For this review, take the finished solid that the model builds, in its own axes (mm). A direction names the side the tool comes from. Round coordinates to 2 decimals unless told otherwise and drop trailing zeros. Write each loop counter-clockwise with the first axis right and the second up, starting at its lowest first coordinate (ties: lowest second). Pieces come first, ordered by that corner, then holes. Notation, with made-up numbers: (57, -37) -> (90, -37) arc R27 ccw to (90, -5) -> close; hole circle Ø8 at (24.5, 70). An arc over 180 degrees is marked (long way). Answer in a Markdown table with one row per item.
from build123d import *

# Parameters (mm, degrees)
F0_R     = 20
F1_DEPTH = 5
F2_R     = 30
F2_R_2   = 20
F3_DEPTH = 5
F4_R     = 30
F4_R_2   = 20
F5_DEPTH = 5


with BuildPart() as f1:
    # F0 (on Top) → F1 (new body)
    with BuildSketch(Plane.XY):
        with BuildLine():
            Line((-160, -90), (160, -90))
            ThreePointArc((160, -90), (174.142136, -84.142136), (180, -70))
            Line((180, -70), (180, 70))
            ThreePointArc((180, 70), (174.142136, 84.142136), (160, 90))
            Line((160, 90), (-160, 90))
            ThreePointArc((-160, 90), (-174.142136, 84.142136), (-180, 70))
            Line((-180, 70), (-180, -70))
            ThreePointArc((-180, -70), (-174.142136, -84.142136), (-160, -90))
        make_face()
        with Locations((-135, -52)):
            Circle(F0_R, mode=Mode.SUBTRACT)
        with Locations((135, -52)):
            Circle(F0_R, mode=Mode.SUBTRACT)
        with Locations((-135, 52)):
            Circle(F0_R, mode=Mode.SUBTRACT)
        with Locations((135, 52)):
            Circle(F0_R, mode=Mode.SUBTRACT)
    extrude(amount=F1_DEPTH)

    # F2 (on face) → F3 (join)
    with BuildSketch(Plane.XY.offset(5)):
        with Locations((-135, 52)):
            Circle(F2_R)
        with Locations((-135, 52)):
            Circle(F2_R_2, mode=Mode.SUBTRACT)
        with Locations((135, 52)):
            Circle(F2_R)
        with Locations((135, 52)):
            Circle(F2_R_2, mode=Mode.SUBTRACT)
        with Locations((-135, -52)):
            Circle(F2_R)
        with Locations((-135, -52)):
            Circle(F2_R_2, mode=Mode.SUBTRACT)
        with Locations((135, -52)):
            Circle(F2_R)
        with Locations((135, -52)):
            Circle(F2_R_2, mode=Mode.SUBTRACT)
    extrude(amount=F3_DEPTH)

    # F4 (on face) → F5 (join)
    with BuildSketch(Plane(origin=(0, 0, 0), x_dir=(1, 0, 0), z_dir=(0, 0, -1))):
        with Locations((-135, 52)):
            Circle(F4_R)
        with Locations((-135, 52)):
            Circle(F4_R_2, mode=Mode.SUBTRACT)
        with Locations((135, 52)):
            Circle(F4_R)
        with Locations((135, 52)):
            Circle(F4_R_2, mode=Mode.SUBTRACT)
        with Locations((-135, -52)):
            Circle(F4_R)
        with Locations((-135, -52)):
            Circle(F4_R_2, mode=Mode.SUBTRACT)
        with Locations((135, -52)):
            Circle(F4_R)
        with Locations((135, -52)):
            Circle(F4_R_2, mode=Mode.SUBTRACT)
    extrude(amount=F5_DEPTH)


solid = f1.part
1) Consider section B-B on y = -52. State the section outline as (x, z) points.
Solved:
| item | result |
|---|---|
| outline | (-180, 0) -> (-165, 0) -> (-165, -5) -> (-155, -5) -> (-155, 10) -> (-165, 10) -> (-165, 5) -> (-180, 5) -> close; (-115, -5) -> (-105, -5) -> (-105, 0) -> (105, 0) -> (105, -5) -> (115, -5) -> (115, 10) -> (105, 10) -> (105, 5) -> (-105, 5) -> (-105, 10) -> (-115, 10) -> close; (155, -5) -> (165, -5) -> (165, 0) -> (180, 0) -> (180, 5) -> (165, 5) -> (165, 10) -> (155, 10) -> close |
2) Clearance check with flat-ended pins moving along their axes: pin 1 Ø1.5 at (x, y) = (102.5, 48) entering from -Z; pin 2 Ø1 at (x, z) = (117, -3) entering from -Y; pin 3 Ø12 at (x, y) = (18, 21.5) entering from +Z. State where each tip first meets the part, or that it passes through.
Solved:
| item | result |
|---|---|
| pin 1 | z = 0 |
| pin 2 | y = -76.37 |
| pin 3 | z = 5 |
3) Consider section C-C on x = 75. State the section outline as (y, z) points.
Solved:
| item | result |
|---|---|
| outline | (-90, 0) -> (90, 0) -> (90, 5) -> (-90, 5) -> close |
4) For faces 1 (the cylindrical face through (115.02, 51.12, 2.61)), 2 (the flat face through (-3, 1, 0)), 3 (the cylindrical face through (111, -70, 7)), list the 3-axis set-ups (+Z, -Z, +X, -X, +Y, -Y) from which the entire face can be reached by the end or side of a thin tool; tool diameter is ignored.
Solved:
| item | result |
|---|---|
| face 1 | +Z, -Z |
| face 2 | -Z |
| face 3 | +Z |
5) Consider section D-D on y = 17. State the section outline as (x, z) points, then the cut area to 3 significant figures.
Solved:
| item | result |
|---|---|
| outline | (-180, 0) -> (180, 0) -> (180, 5) -> (-180, 5) -> close |
| area | 1,800 mm² |
6) For line 1 (Y direction, x = 135, z = 4.5); line 2 (X direction, y = 52, z = 4.75); line 3 (Y direction, x = -135, z = -1.25), list the stretches that pass through material, from the lowest coordinate up. Write a range as [from, to].
Solved:
| item | result |
|---|---|
| line 1 | [-90, -72], [-32, 32], [72, 90] |
| line 2 | [-180, -155], [-115, 115], [155, 180] |
| line 3 | [-82, -72], [-32, -22], [22, 32], [72, 82] |
7) Mouldability with a two-part tool opening along Y and no side actions: class faces 4 (the flat face through (155, 58, -5)), 5 (the cylindrical face through (173.986, -84.297, 2.465)), 6 (the cylindrical face through (111, 34, 7)) as pulls with the +Y half, pulls with the -Y half, needs draft (parallel to the pull), parting line crosses it, or undercut.
Solved:
| item | result |
|---|---|
| face 4 | needs draft |
| face 5 | pulls with the -Y half |
| face 6 | undercut |
8) Consider section A-A on x = -135. State the section outline as (y, z) points.
Solved:
| item | result |
|---|---|
| outline | (-90, 0) -> (-82, 0) -> (-82, -5) -> (-72, -5) -> (-72, 10) -> (-82, 10) -> (-82, 5) -> (-90, 5) -> close; (-32, -5) -> (-22, -5) -> (-22, 0) -> (22, 0) -> (22, -5) -> (32, -5) -> (32, 10) -> (22, 10) -> (22, 5) -> (-22, 5) -> (-22, 10) -> (-32, 10) -> close; (72, -5) -> (82, -5) -> (82, 0) -> (90, 0) -> (90, 5) -> (82, 5) -> (82, 10) -> (72, 10) -> close |
